```python
from build123d import *

# Parameters (mm, degrees)
EXTRUDE_1_DEPTH     = 4
SKETCH_2_R          = 8.2578
CUT_EXTRUDE_1_DEPTH = 242.202090903
SKETCH_3_W          = 12
SKETCH_3_H          = 15
CUT_EXTRUDE_2_DEPTH = 242.202090903
SKETCH_4_R          = 7.273
CUT_EXTRUDE_3_DEPTH = 242.202090903
SKETCH_5_R          = 3.493
CUT_EXTRUDE_4_DEPTH = 242.202090903


with BuildPart() as part:
    # 草图1 → 凸台-拉伸1 (new body)
    with BuildSketch(Plane.XY):
        Polygon((0, 0), (-0.022, 1.356), (0.112, 1.935), (0.273, 2.386), (0.631, 3.114), (1.112, 3.853), (1.618, 4.487), (3.738, 6.498), (5.954, 8.087), (8.221, 9.446), (10.524, 10.652), (16.38, 13.212), (22.333, 15.314), (34.409, 18.579), (46.63, 20.902), (58.933, 22.468), (71.28, 23.384), (83.643, 23.716), (96, 23.519), (108.149, 22.918), (120.282, 22.016), (132.395, 20.844), (144.485, 19.431), (156.547, 17.759), (168.577, 15.85), (180.573, 13.692), (192.529, 11.275), (204.433, 8.534), (216.296, 5.59), (228.111, 2.437), (234.107, 1.62), (240, 0), (234.107, -0.054), (228.111, 0.629), (216.296, 0.276), (204.433, -0.134), (192.529, -0.609), (180.573, -1.026), (168.577, -1.45), (156.547, -1.893), (144.485, -2.365), (132.395, -2.844), (120.282, -3.35), (108.149, -3.852), (96, -4.319), (83.643, -4.816), (71.28, -5.384), (58.933, -5.968), (46.63, -6.502), (34.409, -6.879), (22.333, -6.914), (16.38, -6.687), (10.524, -6.152), (8.221, -5.798), (5.954, -5.315), (3.738, -4.626), (1.618, -3.539), (1.112, -3.14), (0.631, -2.636), (0.273, -2.099), (0.112, -1.743), (-0.022, -1.26), align=None)
    extrude(amount=EXTRUDE_1_DEPTH)

    # 草图2 → 切除-拉伸1 (cut, through all)
    with BuildSketch(Plane.XY):
        with Locations((60, 8.25)):
            Circle(SKETCH_2_R)
    extrude(amount=CUT_EXTRUDE_1_DEPTH, mode=Mode.SUBTRACT)

    # 草图3 → 切除-拉伸2 (cut, through all)
    with BuildSketch(Plane.XY):
        with Locations((96, 17.1)):
            Rectangle(SKETCH_3_W, SKETCH_3_H)
    extrude(amount=CUT_EXTRUDE_2_DEPTH, mode=Mode.SUBTRACT)

    # 草图4 → 切除-拉伸3 (cut, through all)
    with BuildSketch(Plane.XY):
        with Locations((110, 9.5093)):
            Circle(SKETCH_4_R)
    extrude(amount=CUT_EXTRUDE_3_DEPTH, mode=Mode.SUBTRACT)

    # 草图5 → 切除-拉伸4 (cut, through all)
    with BuildSketch(Plane.XY):
        with Locations((160, 7.7037)):
            Circle(SKETCH_5_R)
    extrude(amount=CUT_EXTRUDE_4_DEPTH, mode=Mode.SUBTRACT)


solid = part.part
```
Work out the finished part from the listing and answer in its coordinate system (mm). A direction names the side the tool comes from. Round coordinates to 2 decimals unless told otherwise and drop trailing zeros. Order: outer loops, then holes, each group sorted by start corner. A loop starts at its lowest first (then second) coordinate and runs counter-clockwise, first axis right, second up.
Q1. A cutting plane is placed at B-B, the plane z = 1.3. Count the separate pieces of the cut face and the enclosed holes in it, then the cut area to 3 significant figures.
Solution:
separate pieces: 1
enclosed holes: 3
area: 4,090 mm2
Q2. A cutting plane is placed at A-A, the plane x = 160. Determine the outline of the cut face in (y, z), then the cut area to 3 significant figures.
Solution:
outline: (-1.77, 0) - (4.21, 0) - (4.21, 4) - (-1.77, 4) - close; (11.2, 0) - (17.21, 0) - (17.21, 4) - (11.2, 4) - close
area: 48.0 mm2
Q3. A cutting plane is placed at C-C, the plane x = 124. Determine the outline of the cut face in (y, z), then the cut area to 3 significant figures.
Solution:
outline: (-3.19, 0) - (21.66, 0) - (21.66, 4) - (-3.19, 4) - close
area: 99.4 mm2
Q4. A tool of negligible diameter and unlimited length cuts with its end or side. For faces 1 (the flat face through (90, 17, 2)), 2 (the flat face through (102.16, -4.082, 1.972)), from which of +Z, -Z, +X, -X, +Y, -Y can it reach the whole face along a straight path? Write none if from no direction.
Solution:
face 1: +Z, -Z, +Y
face 2: +Z, -Z, +X, -Y
Q5. The mould has two halves that part along X. Classify faces 3 (the flat face through (95, 5, 4)), 4 (the flat face through (138.355, 20.147, 1.972)), 5 (the flat face through (231.151, 0.283, 1.972)): pulls with the +X half, pulls with the -X half, needs draft (parallel to the pull), parting line crosses it, or undercut.
Solution:
face 3: needs draft
face 4: pulls with the +X half
face 5: undercut
Q6. Find the intervals of material crossed by line 1 along Y through (x, z) = (110, 1.1); line 2 along Y through (x, z) = (160, 3); line 3 along Y through (x, z) = (34.5, 0.45), in increasing order.
Solution:
line 1: y = -3.78 to 2.24, 16.78 to 22.78
line 2: y = -1.77 to 4.21, 11.2 to 17.21
line 3: y = -6.88 to 18.6
